Autodesk Inventor part; units mm, degrees
ref_plane "YZ Plane" through (0, 0, 0) normal (1, 0, 0) x (0, 1, 0)
ref_plane "XZ Plane" through (0, 0, 0) normal (0, 1, 0) x (-1, 0, 0)
ref_plane "XY Plane" through (0, 0, 0) normal (0, 0, 1) x (1, 0, 0)
sketch "Sketch1" plane through (0, 0, 0) normal (0, 1, 0) x (-1, 0, 0)
  circle A0 centre (0, 0) radius 36 construction
  circle A1 centre (0, -50) radius 5
  arc A2 (-9.9499, -49) -> (9.9499, -49) centre (0, -50) ccw
  line L0 (0, 0) -> (0, -50) construction
  line L1 (0, 0) -> (25, -43.3013) construction
  line L2 (0, 0) -> (50, 0) construction
  arc A3 (15.5, -26.8468) -> (20.5, -35.507) centre (18, -31.1769) ccw
  line L3 (0, 0) -> (48.2963, -12.941) construction
  line L4 (0, 0) -> (50, 0) construction
  arc A4 (39.603, -10.6116) -> (29.9437, -8.0234) centre (34.7733, -9.3175) ccw
  arc A5 (29.9437, -8.0234) -> (15.5, -26.8468) centre (0, 0) ccw construction
  arc A6 (39.603, -10.6116) -> (20.5, -35.507) centre (0, 0) ccw construction
  arc A7 (20.5, -35.507) -> (39.603, -10.6116) centre (0, 0) ccw
  arc A8 (15.5, -26.8468) -> (29.9437, -8.0234) centre (0, 0) ccw
  circle A9 centre (-43.3013, -25) radius 5
  arc A10 (-47.4102, -15.8832) -> (-37.4603, -33.1168) centre (-43.3013, -25) ccw
  circle A11 centre (-43.3013, 25) radius 5
  arc A12 (-37.4603, 33.1168) -> (-47.4102, 15.8832) centre (-43.3013, 25) ccw
  circle A13 centre (0, 50) radius 5
  arc A14 (9.9499, 49) -> (-9.9499, 49) centre (0, 50) ccw
  circle A15 centre (43.3013, 25) radius 5
  arc A16 (47.4102, 15.8832) -> (37.4603, 33.1168) centre (43.3013, 25) ccw
  circle A17 centre (43.3013, -25) radius 5
  arc A18 (37.4603, -33.1168) -> (47.4102, -15.8832) centre (43.3013, -25) ccw
  arc A19 (15.5, 26.8468) -> (20.5, 35.507) centre (18, 31.1769) ccw
  arc A20 (20.5, 35.507) -> (-10.6116, 39.603) centre (0, 0) ccw
  arc A21 (15.5, 26.8468) -> (-8.0234, 29.9437) centre (0, 0) ccw
  arc A22 (-10.6116, 39.603) -> (-8.0234, 29.9437) centre (-9.3175, 34.7733) ccw
  arc A23 (-31, 0) -> (-41, 0) centre (-36, 0) ccw
  arc A24 (-41, 0) -> (-28.9914, -28.9914) centre (0, 0) ccw
  arc A25 (-31, 0) -> (-21.9203, -21.9203) centre (0, 0) ccw
  arc A26 (-28.9914, -28.9914) -> (-21.9203, -21.9203) centre (-25.4558, -25.4558) ccw
  arc A27 (9.9499, -49) -> (37.4603, -33.1168) centre (0, 0) ccw
  arc A28 (47.4102, -15.8832) -> (47.4102, 15.8832) centre (0, 0) ccw
  arc A29 (37.4603, 33.1168) -> (9.9499, 49) centre (0, 0) ccw
  arc A30 (-9.9499, 49) -> (-37.4603, 33.1168) centre (0, 0) ccw
  arc A31 (-47.4102, 15.8832) -> (-47.4102, -15.8832) centre (0, 0) ccw
  arc A32 (-37.4603, -33.1168) -> (-9.9499, -49) centre (0, 0) ccw
  circle A33 centre (0, 0) radius 50 construction
  dimension "d20" = 100
  dimension "d0" = 72
  dimension "d4" = 10
  dimension "d5" = 10
  dimension "d6" = 60
  dimension "d7" = 10
  dimension "d8" = 15
  dimension "d10" = 10
  dimension "d13" = 360
  dimension "d17" = 360
  dimension "d19" = 50
extrude "Extrusion1" add sketch "Sketch1" along normal blind 10
properties part number "CE-1.3.2"
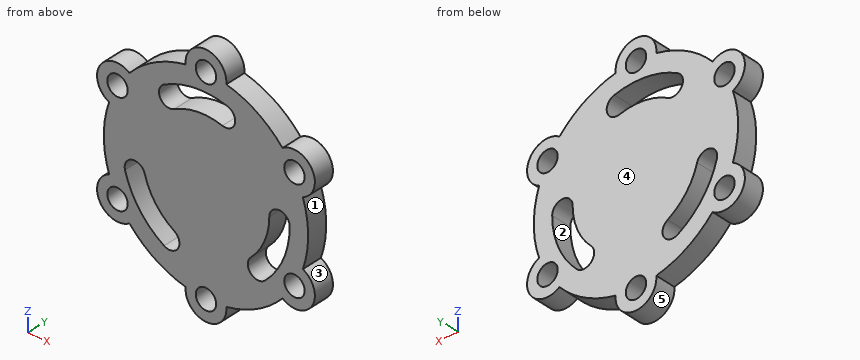
Work out the finished part from the listing and answer in its coordinate system (mm). Face numbers are marked on the shaded views. A direction names the side the tool comes from. Coordinates: 2 decimals unless noted, no trailing zeros. Order: outer loops, then holes, each group sorted by start corner. A loop starts at its lowest first (then second) coordinate and runs counter-clockwise, first axis right, second up. Notation, with made-up numbers: (1.5, 72.5) - (28.5, 72.5) arc R14 ccw to (28.5, 78.5) - close; hole circle Ø4 at (27.25, 22.25). An arc over 180 degrees is marked (long way). Put each result on its own line as item: value. Start each with the question number.
1) Find the intervals of material crossed by line 1 (X direction, y = 2, z = 27); line 2 (Z direction, x = -19.5, y = 3.75); line 3 (X direction, y = 4.5, z = 10), in increasing order. Write a range as from..to.
2) Find section A-A (x = 0). Give the vertices of the cut face in (y, z).
3) Find section B-B (y = 8.5). State how many separate pieces and enclosed holes the cut face has, plus the area to 3 significant figures.
4) Find section D-D (z = -25). Give the vertices of the cut face in (x, y).
5) Flat-ended cylindrical pins translate along their axes: pin 1 (9 mm diameter, centred on x = 0, z = 50, fed in from -Y); pin 2 (1 mm diameter, centred on y = 2.5, z = -31, fed in from +X); pin 3 (3 mm diameter, centred on y = 5, z = 13, fed in from +X); pin 4 (5 mm diameter, centred on y = 2.5, z = -12.5, fed in from -X). Find the tip coordinate at first contact, or state that the pin passes through.
6) Find section C-C (x = 36). Give the vertices of the cut face in (y, z).
7) For a pull along X with two mould halves and no side action, classify the marked faces 3, 4 and 5 as released by +X, released by -X, zero draft, split by the parting line, or undercut.
8) For the marked faces 1 and 2, determine the directions among +Z, -Z, +X, -X, +Y, -Y from which every point of the face is accessible in a straight line to the end or side of a thin tool.
Results list:
1. line 1: x = -53.1..-47.88, -38.72..-20.75, -15.23..38.72, 47.88..53.1
1. line 2: z = -46.04..-35.95, -24.1..26.41, 36.07..46.04
1. line 3: x = -48.99..48.99
2. outline: (0, -60) - (10, -60) - (10, -55) - (0, -55) - close; (0, -45) - (10, -45) - (10, 31) - (0, 31) - close; (0, 41) - (10, 41) - (10, 45) - (0, 45) - close; (0, 55) - (10, 55) - (10, 60) - (0, 60) - close
3. separate pieces: 1
3. enclosed holes: 9
3. area: 7,280 mm^2
4. outline: (-53.3, 0) - (-48.3, 0) - (-48.3, 10) - (-53.3, 10) - close; (-38.3, 0) - (-32.5, 0) - (-32.5, 10) - (-38.3, 10) - close; (-18.33, 0) - (20.48, 0) - (20.48, 10) - (-18.33, 10) - close; (32.5, 0) - (38.3, 0) - (38.3, 10) - (32.5, 10) - close; (48.3, 0) - (53.3, 0) - (53.3, 10) - (48.3, 10) - close
5. pin 1: passes through
5. pin 2: stops at x = 51.65
5. pin 3: stops at x = 48.66
5. pin 4: stops at x = -48.99
6. outline: (0, -34.7) - (10, -34.7) - (10, -19.62) - (0, -19.62) - close; (0, 5) - (10, 5) - (10, 34.7) - (0, 34.7) - close
7. face 3: undercut
7. face 4: zero draft
7. face 5: split by the parting line
8. face 1: +X, +Y, -Y
8. face 2: +Y, -Y
